The listing builds one solid part. Answer for the finished solid, in the listing's coordinates (mm). Face numbers are marked on the shaded views. A direction names the side the tool comes from. Round coordinates to 2 decimals unless told otherwise and drop trailing zeros. Write each loop counter-clockwise with the first axis right and the second up, starting at its lowest first coordinate (ties: lowest second). Pieces come first, ordered by that corner, then holes.
Item 1: Find section A-A on y = -86.5. Give the vertices of the cut face in (x, z), then the cut area to 3 significant figures.
Item 2: Find section B-B on z = 566. Give the vertices of the cut face in (x, y), then the cut area to 3 significant figures.
Item 3: Find the intervals of material crossed by probe 1 along Y at (x, z) = (33.5, 425.5); probe 2 along Z at (x, y) = (508, -211.5); probe 3 along Z at (x, y) = (424.5, -357.5), in increasing order.
Item 4: For a pull along X with two mould halves and no side action, classify the marked faces 4, 5, 6 and 7 as +X half, -X half, draft (parallel to the pull), parting line (faces both ways), or undercut.
Item 5: A tool of negligible diameter and unlimited length cuts with its end or side. For the marked faces 1, 2 and 3, from which of +Z, -Z, +X, -X, +Y, -Y can it reach the whole face along a straight path? Write none if from no direction.
Item 6: Find section D-D on x = 493.5. Give the vertices of the cut face in (y, z).
Item 7: Find section C-C on x = 202. Give the vertices of the cut face in (y, z), then the cut area to 3 significant figures.
Item 8: Each of these flat-tipped pins is pushed along its axis until it touches: pin 1 (4 mm diameter, centred on x = 162, z = 668.5, fed in from -Y); pin 2 (2 mm diameter, centred on x = 263.5, y = -441.5, fed in from +Z); pin 3 (12 mm diameter, centred on x = 425.5, y = -574, fed in from +Z). Where does it stop, or does it pass through?
```python
from build123d import *

# Parameters (mm, degrees)
F1_DEPTH = 1000
F0_W     = 320
F0_H     = 160
F2_DEPTH = 150
F3_W     = 120
F3_H     = 400
F4_DEPTH = 700
F6_DEPTH = 267.208


with BuildPart() as f1:
    # F0 (on Front) → F1 (new body)
    with BuildSketch(Plane.XZ):
        Polygon((0, 220), (0, 0), (238.846631, 0), (170, 119.245863), (470, 119.245863), (401.153369, 0), (640, 0), (640, 220), align=None)
    extrude(amount=F1_DEPTH)

    # F0 (on Front) → F2 (join)
    with BuildSketch(Plane.XZ):
        Polygon((0, 620), (0, 220), (640, 220), (640, 620), (480, 620), (160, 620), align=None)
        Polygon((480, 620), (640, 620), (480, 780), align=None)
        with Locations((320, 700)):
            Rectangle(F0_W, F0_H)
        Polygon((160, 780), (0, 620), (160, 620), align=None)
    extrude(amount=F2_DEPTH)

    # F3 (on face) → F4 (join)
    with BuildSketch(Plane.XZ.offset(150)):
        with Locations((320, 420)):
            Rectangle(F3_W, F3_H)
    extrude(amount=F4_DEPTH)

    # F5 (on face) → F6 (cut)
    with BuildSketch(Plane.YZ.offset(380)):
        Polygon((-850, 620), (-850, 220), (-150, 620), align=None)
    extrude(amount=-F6_DEPTH, mode=Mode.SUBTRACT)


solid = f1.part
```
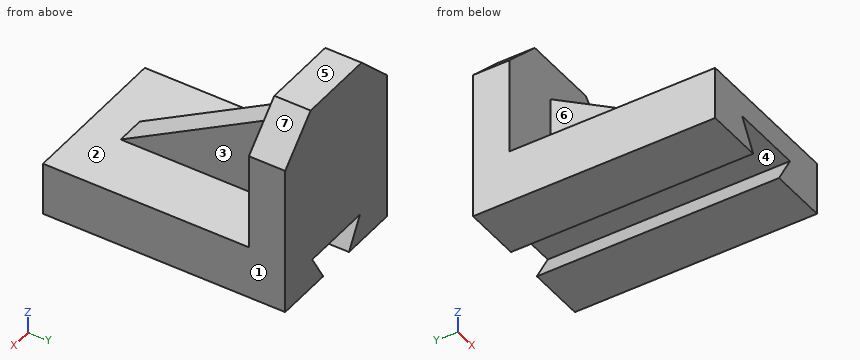
Check values:
1. outline: (0, 0) - (238.85, 0) - (170, 119.25) - (470, 119.25) - (401.15, 0) - (640, 0) - (640, 620) - (480, 780) - (160, 780) - (0, 620) - close
1. area: 446,000 mm2
2. outline: (0, -150) - (260, -150) - (260, -244.5) - (380, -244.5) - (380, -150) - (640, -150) - (640, 0) - (0, 0) - close
2. area: 107,000 mm2
3. probe 1: y = -150 to 0
3. probe 2: z = 0 to 220
3. probe 3: z = 0 to 40.44, 119.25 to 220
4. face 4: undercut
4. face 5: draft
4. face 6: -X half
4. face 7: +X half
5. face 1: +Z, -Z, +X, +Y, -Y
5. face 2: +Z, -Y
5. face 3: +Z, +X, -Y
6. outline: (-1000, 0) - (0, 0) - (0, 766.5) - (-150, 766.5) - (-150, 220) - (-1000, 220) - close
7. outline: (-1000, 0) - (0, 0) - (0, 63.82) - (-1000, 63.82) - close; (-1000, 119.25) - (0, 119.25) - (0, 780) - (-150, 780) - (-150, 220) - (-1000, 220) - close
7. area: 249,000 mm2
8. pin 1: stops at y = -150
8. pin 2: stops at z = 454
8. pin 3: stops at z = 220
